Read the model definition and answer for the solid it produces. Units are mm, in the model's axes. A direction names the side the tool comes from. Coordinates: 2 decimals unless noted, no trailing zeros. Order: outer loops, then holes, each group sorted by start corner. A loop starts at its lowest first (then second) coordinate and runs counter-clockwise, first axis right, second up. Notation, with made-up numbers: (44, 5.25) -> (94, 5.25) arc R25 ccw to (94, 36.25) -> close; hole circle Ø6 at (89.25, -38). An arc over 180 degrees is marked (long way). Answer as a JSON object with one key per item and string values. Group by question number.
1) Consider L1, parallel to Y at x = 251.5, z = -18.5; L2, parallel to Y at x = 254, z = 77.5; L3, parallel to Z at x = -320.5, y = 79. Determine where each line is inside the solid, lowest interval first.
2) Section B-B on x = 254 is taken. Determine the outline of the cut face in (y, z).
3) Section A-A on y = 50.8 is taken. Determine the outline of the cut face in (x, z).
4) Determine the mould class of faces 1 (the flat face through (-482.6, 50, 3)), 2 (the flat face through (0, 50, 254)), 3 (the flat face through (-152.4, 52, -190)), 4 (the flat face through (-114, 101.6, -4)) for opening direction Z: released by +Z, released by -Z, zero draft, split by the parting line, or undercut.
5) A tool of negligible diameter and unlimited length cuts with its end or side. For faces 5 (the flat face through (303, 164, -241.3)), 6 (the flat face through (266, 158, 228.6)), 7 (the flat face through (431.8, 127, 3)), 8 (the flat face through (-355.6, 52, 191)), from which of +Z, -Z, +X, -X, +Y, -Y can it reach the whole face along a straight path? Write none if from no direction.
6) Given pin 1 (10 mm diameter, centred on x = -183, z = -54.5, fed in from +Y); pin 2 (6 mm diameter, centred on x = 385, z = -17, fed in from +Y); pin 3 (6 mm diameter, centred on x = 385.5, y = 128, fed in from -Z), each flat-ended and moving along its own axis, determine where each tip first touches the part or whether it passes through.
7) Section C-C on z = -194 is taken. Determine the outline of the cut face in (x, y), and give its area (3 significant figures).
8) Section D-D on x = -254 is taken. Determine the outline of the cut face in (y, z).
from build123d import *

# Parameters (mm, degrees)
SKETCH1_W           = 965.2
SKETCH1_H           = 508
BOSS_EXTRUDE1_DEPTH = 101.6
SKETCH2_R           = 21.59
CUT_EXTRUDE1_DEPTH  = 509
FILLET1_R           = 38.1
FILLET2_R           = 25.4
CUT_EXTRUDE2_REACH  = 103.6
SKETCH4_W           = 203.2
SKETCH4_H           = 25.4
SKETCH6_W           = 253.917216802
SKETCH6_H           = 482.6
BOSS_EXTRUDE3_DEPTH = 127
FILLET4_R           = 76.2
SKETCH7_W           = 457.2
SKETCH7_H           = 114.3
CUT_EXTRUDE4_DEPTH  = 179


with BuildPart() as part:
    # Sketch1 → Boss-Extrude1 (new body)
    with BuildSketch(Plane(origin=(0, 0, 0), x_dir=(1, 0, 0), z_dir=(0, 1, 0))):
        Rectangle(SKETCH1_W, SKETCH1_H)
    extrude(amount=BOSS_EXTRUDE1_DEPTH)

    # Sketch2 → Cut-Extrude1 (cut, through all)
    with BuildSketch(Plane.XY.offset(254)):
        with Locations((254, 50.8)):
            Circle(SKETCH2_R)
    extrude(amount=-CUT_EXTRUDE1_DEPTH, mode=Mode.SUBTRACT)

    # Fillet1
    fillet1_edges = [part.edges().sort_by_distance(p)[0] for p in [
        (-482.6, 50.8, -254),
        (-482.6, 50.8, 254),
    ]]
    fillet(fillet1_edges, radius=FILLET1_R)

    # Fillet2
    fillet2_edges = [part.edges().sort_by_distance(p)[0] for p in [
        (482.6, 50.8, -254),
        (482.6, 50.8, 254),
    ]]
    fillet(fillet2_edges, radius=FILLET2_R)

    # Sketch4 → Cut-Extrude2 (cut, up to next)
    with BuildSketch(Plane(origin=(0, 101.6, 0), x_dir=(1, 0, 0), z_dir=(0, 1, 0)), mode=Mode.PRIVATE) as cut_extrude2_sk1:
        with Locations((-254, -190.5)):
            Rectangle(SKETCH4_W, SKETCH4_H)
    cut_extrude2_tool1 = extrude(cut_extrude2_sk1.sketch, amount=-CUT_EXTRUDE2_REACH, mode=Mode.PRIVATE) & part.part
    add(cut_extrude2_tool1.solids().sort_by_distance((-254, 101.6, 190.5))[0], mode=Mode.SUBTRACT)
    # Sketch4 → Cut-Extrude2 (cut, up to next)
    with BuildSketch(Plane(origin=(0, 101.6, 0), x_dir=(1, 0, 0), z_dir=(0, 1, 0)), mode=Mode.PRIVATE) as cut_extrude2_sk2:
        with Locations((-254, 190.5)):
            Rectangle(SKETCH4_W, SKETCH4_H)
    cut_extrude2_tool2 = extrude(cut_extrude2_sk2.sketch, amount=-CUT_EXTRUDE2_REACH, mode=Mode.PRIVATE) & part.part
    add(cut_extrude2_tool2.solids().sort_by_distance((-254, 101.6, -190.5))[0], mode=Mode.SUBTRACT)

    # Sketch6 → Boss-Extrude3 (add)
    with BuildSketch(Plane(origin=(0, 101.6, 0), x_dir=(1, 0, 0), z_dir=(0, 1, 0))):
        with Locations((304.841391599, 0)):
            Rectangle(SKETCH6_W, SKETCH6_H)
    extrude(amount=BOSS_EXTRUDE3_DEPTH)

    # Fillet4
    fillet4_edges = [part.edges().sort_by_distance(p)[0] for p in [
        (431.8, 228.6, 0),
    ]]
    fillet(fillet4_edges, radius=FILLET4_R)

    # Sketch7 → Cut-Extrude4 (cut)
    with BuildSketch(Plane.ZY.offset(-177.882783198)):
        with Locations((0, 158.75)):
            Rectangle(SKETCH7_W, SKETCH7_H)
    extrude(amount=-CUT_EXTRUDE4_DEPTH, mode=Mode.SUBTRACT)


solid = part.part
Worked answers:
{
 "1": {"L1": "y = 0 to 29.36, 72.24 to 101.6, 215.9 to 228.6", "L2": "y = 0 to 29.21, 72.39 to 101.6, 215.9 to 228.6", "L3": "z = -254 to -203.2, -177.8 to 177.8, 203.2 to 254"},
 "2": {"outline": "(0, -254) -> (29.21, -254) -> (29.21, 254) -> (0, 254) -> close; (72.39, -254) -> (101.6, -254) -> (101.6, -241.3) -> (228.6, -241.3) -> (228.6, 241.3) -> (101.6, 241.3) -> (101.6, 254) -> (72.39, 254) -> close; hole (101.6, -228.6) -> (215.9, -228.6) -> (215.9, 228.6) -> (101.6, 228.6) -> close"},
 "3": {"outline": "(-482.6, -215.9) arc R38.1 ccw to (-444.5, -254) -> (232.41, -254) -> (232.41, 254) -> (-444.5, 254) arc R38.1 ccw to (-482.6, 215.9) -> close; (275.59, -254) -> (457.2, -254) arc R25.4 ccw to (482.6, -228.6) -> (482.6, 228.6) arc R25.4 ccw to (457.2, 254) -> (275.59, 254) -> close; hole (-355.6, -203.2) -> (-152.4, -203.2) -> (-152.4, -177.8) -> (-355.6, -177.8) -> close; hole (-355.6, 177.8) -> (-152.4, 177.8) -> (-152.4, 203.2) -> (-355.6, 203.2) -> close"},
 "4": {"face 1": "zero draft", "face 2": "released by +Z", "face 3": "undercut", "face 4": "undercut"},
 "5": {"face 5": "-Z, +X, -X, +Y", "face 6": "-X", "face 7": "+Z, -Z, +X, +Y", "face 8": "+Y, -Y"},
 "6": {"pin 1": "stops at y = 101.6", "pin 2": "stops at y = 223.88", "pin 3": "stops at z = -241.3"},
 "7": {"outline": "(-482.6, 0) -> (-355.6, 0) -> (-355.6, 101.6) -> (-482.6, 101.6) -> close; (-152.4, 0) -> (482.6, 0) -> (482.6, 101.6) -> (431.8, 101.6) -> (431.8, 152.4) arc R76.2 ccw to (355.6, 228.6) -> (177.88, 228.6) -> (177.88, 215.9) -> (356.88, 215.9) -> (356.88, 101.6) -> (-152.4, 101.6) -> close; hole circle Ø43.18 at (254, 50.8)", "area": "86,500 mm²"},
 "8": {"outline": "(0, -254) -> (101.6, -254) -> (101.6, -203.2) -> (0, -203.2) -> close; (0, -177.8) -> (101.6, -177.8) -> (101.6, 177.8) -> (0, 177.8) -> close; (0, 203.2) -> (101.6, 203.2) -> (101.6, 254) -> (0, 254) -> close"}
}
